Verification items for this drawing (mm, ordinates from the low corner). A direction names the side the tool comes from. Give positions to 0.01 mm unless a question says otherwise; leave off trailing zeros. Order: outer loops, then holes, each group sorted by start corner. A loop starts at its lowest first (then second) coordinate and runs counter-clockwise, first axis right, second up. Notation, with made-up numbers: M 6,35.5 L 42,35.5 A13 ccw 42,55.5 Z; hole C 52,-8 d4. An arc over 180 degrees is marked long. Return JSON: item names as keys, results as strings. Group by question number.
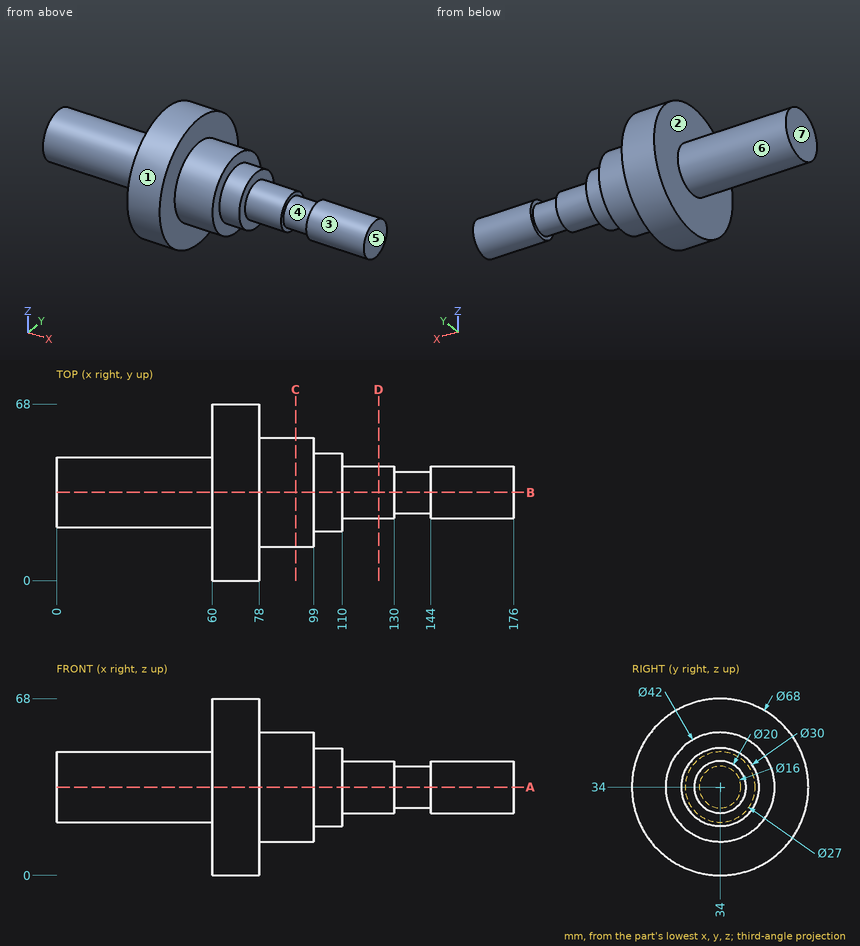
1) Release check for a two-part mould opening along X. For the marked faces 4, 5, 6 and 7 record: released by +X, released by -X, zero draft, split by the parting line, or undercut.
2) Material ranges on line 1 along X through (y, z) = (21.5, 13); line 2 along X through (y, z) = (49, 25.5); line 3 along Z through (x, y) = (67.5, 35.5), recorded low to high.
3) Depth check by flat-ended pin: P1, Ø3, axis at y = 43.5, z = 17, coming from the -X side; P2, Ø5, axis at x = 38.5, z = 29, coming from the +Y side; P3, Ø5, axis at y = 28.5, z = 57.5, coming from the +X side; P4, Ø20.5, axis at y = 40, z = 46, coming from the -X side. Enter the tip coordinate at first touch or a pass-through.
4) Sectioned sample at C-C on x = 92. Record the boundary of the cut face in (y, z).
5) Tool access check on the marked faces 1, 2 and 3. Record the directions out of +Z, -Z, +X, -X, +Y, -Y that give a thin tool (end or side, any length) a straight path to the whole face; none if there is none.
6) Sectioned sample at A-A on z = 34. Record the boundary of the cut face in (x, y).
7) Sectioned sample at D-D on x = 124. Record the boundary of the cut face in (y, z).
Reply:
{
 "1": {"face 4": "undercut", "face 5": "released by +X", "face 6": "zero draft", "face 7": "released by -X"},
 "2": {"line 1": "60 to 78", "line 2": "60 to 99", "line 3": "0.03 to 67.97"},
 "3": {"P1": "x = 60", "P2": "y = 47.27", "P3": "x = 78", "P4": "x = 0"},
 "4": {"outline": "C 34,34 d42"},
 "5": {"face 1": "+X, -X", "face 2": "-X", "face 3": "+X"},
 "6": {"outline": "M 0,20.5 L 60,20.5 L 60,0 L 78,0 L 78,13 L 99,13 L 99,19 L 110,19 L 110,24 L 130,24 L 130,26 L 144,26 L 144,24 L 176,24 L 176,44 L 144,44 L 144,42 L 130,42 L 130,44 L 110,44 L 110,49 L 99,49 L 99,55 L 78,55 L 78,68 L 60,68 L 60,47.5 L 0,47.5 Z"},
 "7": {"outline": "C 34,34 d20"}
}
